Here's how the part is built. I have some questions about the finished solid (model axes, mm). A direction names the side the tool comes from. Round coordinates to 2 decimals unless told otherwise and drop trailing zeros. Write each loop counter-clockwise with the first axis right and the second up, starting at its lowest first coordinate (ties: lowest second). Pieces come first, ordered by that corner, then holes. Notation, with made-up numbers: M 9.5,50.5 L 54.5,50.5 A24 cw 54.5,86.5 Z; hole C -17,-8.5 d5. An arc over 180 degrees is marked long. Write item = value, one per line. Start each with the question number.
(1) If we mould it in two halves opening along Z, with no side actions, what happens to faces 1 (the cylindrical face through (-9.76, 50.31, -2.17)), 2 (the cylindrical face through (-5.361, -17.745, 0.07)), 3 (the flat face through (0, 2, 0))? For each: released by +Z, released by -Z, zero draft, split by the parting line, or undercut.
(2) On a 3-axis mill with a long thin cutter (end or side, diameter ignored), from which of +Z, -Z, +X, -X, +Y, -Y can I reach the whole of each face in a straight line? I mean faces 4 (the cylindrical face through (-7.81, 50.31, -1.73)), 5 (the flat face through (0, 0, 6)), 6 (the flat face through (0, 0, -6)), 7 (the flat face through (8.2, 100, 0)). Say none if no direction works.
(3) Will these pins go through, and if not, where does the flat tip stop? pin 1 Ø4 at (x, y) = (-7.5, -3.5) entering from +Z; pin 2 Ø5 at (x, z) = (-4, 1) entering from +Y; pin 3 Ø2.5 at (x, z) = (2.5, 6) entering from -Y.
(4) I want a section at A-A (y = -10). List the corners of the cut face in (x, z) for me.
(5) I need wall thicknesses on line 1 along X through (y, z) = (71.5, 0); line 2 along Y through (x, z) = (0, 2.75); line 3 along X through (y, z) = (-3, -0.75). Which ranges of each line are inside material? Lowest first, please.
(6) I want a section at C-C (y = 76). List the corners of the cut face in (x, z) for me.
```python
from build123d import *

# Parameters (mm, degrees)
SKETCH1_R                = 10
BOSS_EXTRUDE1_DEPTH      = 100
SHELL1_T                 = -2
FILLET1_R                = 2
BOSS_EXTRUDE2_DEPTH      = 20
BOSS_EXTRUDE2_DEPTH_BACK = 1
SKETCH2_W                = 15
SKETCH2_H                = 10
SKETCH3_R                = 5
CUT_EXTRUDE1_DEPTH       = 20
FILLET2_R                = 7.5


with BuildPart() as part:
    # Sketch1 → Boss-Extrude1 (new body)
    with BuildSketch(Plane(origin=(0, 0, 0), x_dir=(1, 0, 0), z_dir=(0, 1, 0))):
        with Locations(Location((0, 0, 0), (0, 0, 270))):
            Circle(SKETCH1_R)
    extrude(amount=BOSS_EXTRUDE1_DEPTH)

    # Shell1
    shell1_openings = [part.faces().sort_by_distance(p)[0] for p in [
        (0, 100, 0),
    ]]
    offset(amount=SHELL1_T, openings=shell1_openings, kind=Kind.INTERSECTION)

    # Fillet1
    fillet1_edges = [part.edges().sort_by_distance(p)[0] for p in [
        (0, 0, -10),
    ]]
    fillet(fillet1_edges, radius=FILLET1_R)

    # Sketch2 → Boss-Extrude2 (add, two sides: drawn at the far end of the back side and taken through both)
    with BuildSketch(Plane.XZ.offset(-BOSS_EXTRUDE2_DEPTH_BACK)):
        Rectangle(SKETCH2_W, SKETCH2_H)
    extrude(amount=BOSS_EXTRUDE2_DEPTH + BOSS_EXTRUDE2_DEPTH_BACK)

    # Sketch3 → Cut-Extrude1 (cut)
    with BuildSketch(Plane.XY.offset(5)):
        with Locations((0, -10)):
            Circle(SKETCH3_R)
    extrude(amount=-CUT_EXTRUDE1_DEPTH, mode=Mode.SUBTRACT)

    # Fillet2
    fillet2_edges = [part.edges().sort_by_distance(p)[0] for p in [
        (7.5, -20, 0),
        (-7.5, -20, 0),
    ]]
    fillet(fillet2_edges, radius=FILLET2_R - 0.0001)  # a hair under: the kernel refuses the full size


solid = part.part
```
Returned:
q1.face_1 = split by the parting line
q1.face_2 = zero draft
q1.face_3 = undercut
q2.face_4 = +Y
q2.face_5 = +Z, +X, -X, -Y
q2.face_6 = -Z, +X, -X, -Y
q2.face_7 = +Z, -Z, +X, -X, +Y
q3.pin_1 = 5
q3.pin_2 = 2
q3.pin_3 = -19.79
q4.outline = M -7.5,-5 L -5,-5 L -5,5 L -7.5,5 Z; M 5,-5 L 7.5,-5 L 7.5,5 L 5,5 Z
q5.line_1 = -10 to -8, 8 to 10
q5.line_2 = -20 to -15, -5 to 2
q5.line_3 = -7.5 to 7.5
q6.outline = C 0,0 d20; hole C 0,0 d16
